Design review of the part shown in the three views and the two pictorial views. Dimensions are in mm from the part's minimum x, y and z. Give positions to 0.01 mm unless a question says otherwise; leave off trailing zeros. Loops run counter-clockwise (first coordinate to the right, second up) from the corner with the lowest first, then second, coordinate; pieces in that order, holes last. Notation, with made-up numbers: (72.5, 50.5) - (96.5, 50.5) arc R25 ccw to (96.5, 75.5) - close; hole circle Ø1 at (50, -13). An arc over 180 degrees is marked (long way). Use CSV: the item, a comma, the result in double quotes. Start each with the question number.
1. Wall thickness on line 1 (Y direction, x = 8.5, z = 2.5); line 2 (Y direction, x = 8, z = 1.7); line 3 (X direction, y = 20, z = 1.7): over which ranges is each line inside the solid? List them lowest first.
2. Take a section at B-B on y = 21. Give the boundary of the cut face in (x, z).
3. Take a section at A-A on z = 1.95. State how many separate pieces and enclosed holes the cut face has, plus the area to 3 significant figures.
4. For pin 1 (3 mm diameter, centred on x = 8, y = 33, fed in from -Z), flat-tipped, find the tip position at first contact; note if it passes through.
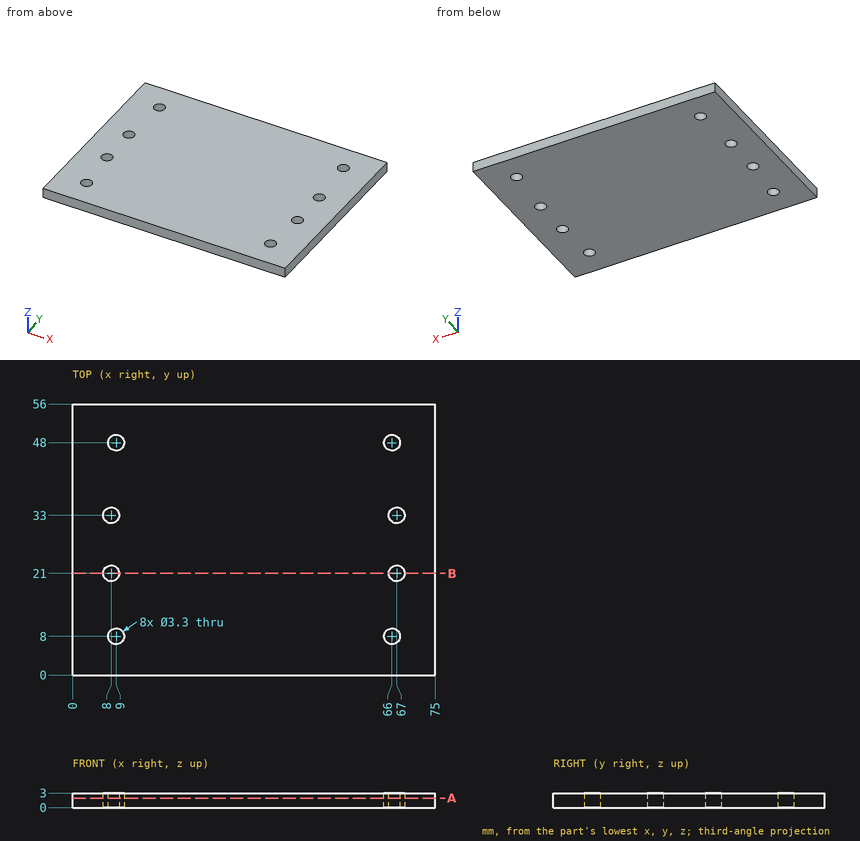
Check result:
1,line 1,"y = 0 to 6.43, 9.57 to 19.43, 22.57 to 31.43, 34.57 to 46.43, 49.57 to 56"
1,line 2,"y = 0 to 6.69, 9.31 to 19.35, 22.65 to 31.35, 34.65 to 46.69, 49.31 to 56"
1,line 3,"x = 0 to 6.69, 9.31 to 65.69, 68.31 to 75"
2,outline,"(0, 0) - (6.35, 0) - (6.35, 3) - (0, 3) - close; (9.65, 0) - (65.35, 0) - (65.35, 3) - (9.65, 3) - close; (68.65, 0) - (75, 0) - (75, 3) - (68.65, 3) - close"
3,separate pieces,"1"
3,enclosed holes,"8"
3,area,"4,130 mm²"
4,pin 1,"passes through"
